For this review, use the dimensioned drawing (mm, ordinates from the lowest corner) and the shaded views. A direction names the side the tool comes from. Give positions to 0.01 mm unless a question says otherwise; leave off trailing zeros. Order: outer loops, then holes, each group sorted by start corner. A loop starts at its lowest first (then second) coordinate and runs counter-clockwise, first axis right, second up.
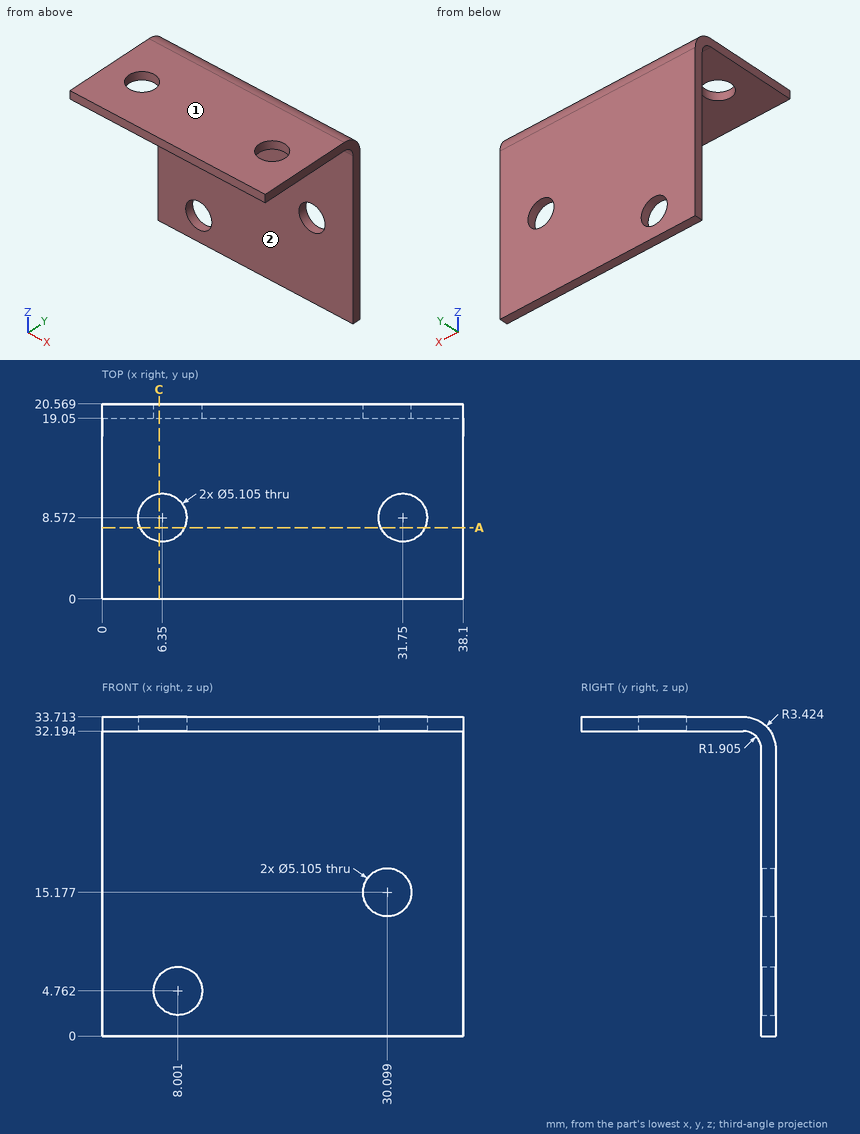
1. Insertion check: pin 1 (10 mm diameter, centred on x = 8.5, y = 6.5, fed in from -Z) (1 decimal); pin 2 (8 mm diameter, centred on x = 32, z = 7, fed in from -Y). Each pin has a flat end and moves straight along its axis. Give the tip position at first contact, or say it passes through.
2. Take a section at C-C (x = 6). Count the separate pieces of the cut face and the enclosed holes in it.
3. Take a section at A-A (y = 7.5). Write out the cut boundary in (x, z) (1 decimal).
4. For the marked faces 1 and 2, list the 3-axis set-ups (+Z, -Z, +X, -X, +Y, -Y) from which the entire face can be reached by the end or side of a thin tool; tool diameter is ignored.
5. To check wall thickness, follow line 1 (Y direction, x = 22.5, z = 6.5); line 2 (Z direction, x = 27, y = 4) (1 decimal); line 3 (Y direction, x = 6.35, z = 32.75) (1 decimal). State the ranges of each line that lie inside material, in increasing order.
Answer:
1. pin 1: stops at z = 32.2
1. pin 2: stops at y = 19.05
2. separate pieces: 3
2. enclosed holes: 0
3. outline: (0, 32.2) - (4, 32.2) - (4, 33.7) - (0, 33.7) - close; (8.7, 32.2) - (29.4, 32.2) - (29.4, 33.7) - (8.7, 33.7) - close; (34.1, 32.2) - (38.1, 32.2) - (38.1, 33.7) - (34.1, 33.7) - close
4. face 1: +Z, +X, -X, +Y, -Y
4. face 2: -Z, +X, -X, -Y
5. line 1: y = 19.05 to 20.57
5. line 2: z = 32.2 to 33.7
5. line 3: y = 0 to 6, 11.1 to 19.5
